Part model, mm, in its own coordinate system. Face numbers are marked on the shaded views. A direction names the side the tool comes from. Give positions to 0.01 mm unless a question says otherwise; leave off trailing zeros. Write each loop counter-clockwise with the first axis right and the second up, starting at its lowest first coordinate (ties: lowest second). Pieces come first, ordered by that corner, then holes. Notation, with made-up numbers: M 80.25,-24 L 136.25,-24 A18 cw 136.25,11 Z; hole C -13,13.25 d5. An arc over 180 degrees is marked long. Use a Markdown table: item, result. Add a question column.
from build123d import *

# Parameters (mm, degrees)
SKETCH_1_R          = 2.5
EXTRUDE_1_DEPTH     = 10
SKETCH_2_R          = 4.5
CUT_EXTRUDE_2_DEPTH = 20


with BuildPart() as part:
    # 草圖1 → 填料-伸長1 (new body)
    with BuildSketch(Plane.XY):
        Polygon((0, 0), (0, 15), (10, 15), (10, 10), (30, 10), (30, 0), align=None)
        with Locations((5, 5)):
            Circle(SKETCH_1_R, mode=Mode.SUBTRACT)
        with Locations((20, 5)):
            Circle(SKETCH_1_R, mode=Mode.SUBTRACT)
    extrude(amount=EXTRUDE_1_DEPTH)

    # 草圖2 → 除料-伸長2 (cut)
    with BuildSketch(Plane(origin=(30, 0, 0), x_dir=(0, 0, -1), z_dir=(1, 0, 0))):
        with Locations((-5, 12.25)):
            Circle(SKETCH_2_R)
    extrude(amount=-CUT_EXTRUDE_2_DEPTH, mode=Mode.SUBTRACT)


solid = part.part
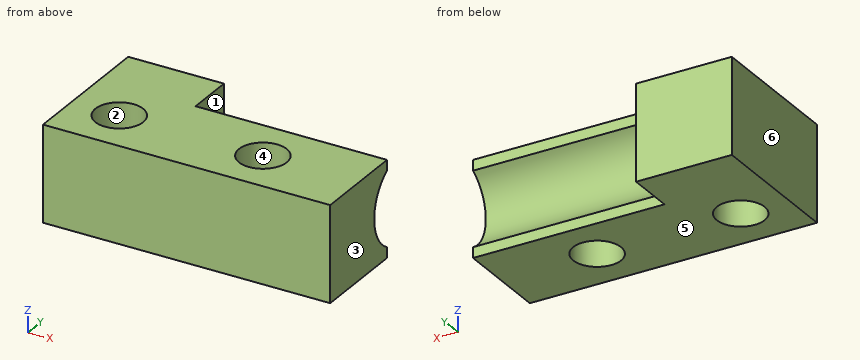
1. Tool access for the marked faces 1 and 2: list every direction of +Z, -Z, +X, -X, +Y, -Y with a clear straight run to the whole face (end or side of a thin tool).
2. Flat gauge pins, fed straight in: pin 1 (0.6 mm diameter, centred on x = 21, z = 0.5, fed in from +Y); pin 2 (6 mm diameter, centred on y = 12.5, z = 3, fed in from +X). Where does each tip first touch, or does it go through?
3. Cut at A-A (x = 5). Write the cut outline in (y, z), then the cut area to 3 significant figures.
4. Cut at C-C (x = 23.75). Write the cut outline in (y, z), then the cut area to 3 significant figures.
5. Drill centre lines: probe 1 along Y at (x, z) = (5, 7.25); probe 2 along X at (y, z) = (4, 9.75); probe 3 along X at (y, z) = (4.75, 8.5). Where is each one in solid material? Low to high. Write a range as [from, to].
6. Cut at B-B (y = 5). Write the cut outline in (x, z), then the cut area to 3 significant figures.
7. Mould opens along X. For the marked faces 3, 4, 5 and 6 say: released by +X, released by -X, zero draft, split by the parting line, or undercut.
8. Cut at D-D (z = 7). Write the cut outline in (x, y), then the cut area to 3 significant figures.
A:
| question | item | result |
|---|---|---|
| 1 | face 1 | +X, +Y |
| 1 | face 2 | +Z, -Z |
| 2 | pin 1 | stops at y = 10 |
| 2 | pin 2 | stops at x = 10 |
| 3 | outline | M 0,0 L 2.5,0 L 2.5,10 L 0,10 Z; M 7.5,0 L 15,0 L 15,10 L 7.5,10 Z |
| 3 | area | 100 mm² |
| 4 | outline | M 0,0 L 10,0 L 10,1.1 A4.5 cw 10,8.9 L 10,10 L 0,10 Z |
| 4 | area | 87.6 mm² |
| 5 | probe 1 | y = [0, 2.5], [7.5, 15] |
| 5 | probe 2 | x = [0, 2.71], [7.29, 17.71], [22.29, 30] |
| 5 | probe 3 | x = [0, 2.51], [7.49, 17.51], [22.49, 30] |
| 6 | outline | M 0,0 L 2.5,0 L 2.5,10 L 0,10 Z; M 7.5,0 L 17.5,0 L 17.5,10 L 7.5,10 Z; M 22.5,0 L 30,0 L 30,10 L 22.5,10 Z |
| 6 | area | 200 mm² |
| 7 | face 3 | released by +X |
| 7 | face 4 | undercut |
| 7 | face 5 | zero draft |
| 7 | face 6 | released by -X |
| 8 | outline | M 0,0 L 30,0 L 30,8.22 L 10,8.22 L 10,15 L 0,15 Z; hole C 5,5 d5; hole C 20,5 d5 |
| 8 | area | 275 mm² |
